from build123d import *

# Parameters (mm, degrees)
SKETCH1_W           = 10
SKETCH1_H           = 25
BOSS_EXTRUDE1_DEPTH = 8
SKETCH8_W           = 10
SKETCH8_H           = 2.3
BOSS_EXTRUDE4_DEPTH = 4
SKETCH9_W           = 10
SKETCH9_H           = 0.2
CUT_EXTRUDE3_DEPTH  = 4
SKETCH4_R           = 1.475
CUT_EXTRUDE2_DEPTH  = 8
LPATTERN1_COUNT     = 4
LPATTERN1_PITCH     = 5


with BuildPart() as part:
    # Sketch1 → Boss-Extrude1 (new body)
    with BuildSketch(Plane(origin=(0, 0, 0), x_dir=(1, 0, 0), z_dir=(0, 1, 0))):
        Rectangle(SKETCH1_W, SKETCH1_H)
    extrude(amount=BOSS_EXTRUDE1_DEPTH)

    # Sketch8 → Boss-Extrude4 (add)
    with BuildSketch(Plane(origin=(0, 8, 0), x_dir=(1, 0, 0), z_dir=(0, 1, 0))):
        with Locations((0, 11.35)):
            Rectangle(SKETCH8_W, SKETCH8_H)
        with Locations((0, -11.35)):
            Rectangle(SKETCH8_W, SKETCH8_H)
    extrude(amount=BOSS_EXTRUDE4_DEPTH)

    # Sketch9 → Cut-Extrude3 (cut)
    with BuildSketch(Plane(origin=(0, 8, 0), x_dir=(1, 0, 0), z_dir=(0, 1, 0))):
        with Locations((0, 10.1)):
            Rectangle(SKETCH9_W, SKETCH9_H)
        with Locations((0, -10.1)):
            Rectangle(SKETCH9_W, SKETCH9_H)
    extrude(amount=-CUT_EXTRUDE3_DEPTH, mode=Mode.SUBTRACT)

    # Sketch4 → Cut-Extrude2 (cut)
    with BuildSketch(Plane.XZ):
        with Locations(Location((0, 7.5, 0), (0, 0, 270))):
            Circle(SKETCH4_R)
    cut_extrude2 = extrude(amount=-CUT_EXTRUDE2_DEPTH, mode=Mode.SUBTRACT)

    # LPattern1: Cut-Extrude2 ×4
    with Locations(*[(0, 0, -i * LPATTERN1_PITCH) for i in range(1, LPATTERN1_COUNT)]):
        add(cut_extrude2, mode=Mode.SUBTRACT)


solid = part.part
CAD build for the part. Positions are in the model's coordinates, mm. A direction names the side the tool comes from. Round coordinates to 2 decimals unless told otherwise and drop trailing zeros. Loops run counter-clockwise (first coordinate to the right, second up) from the corner with the lowest first, then second, coordinate; pieces in that order, holes last.
(1) Cut at A-A (y = 7.5). Give the cut face in (x, z) (3 decimals).
(2) Cut at B-B (z = 2.5). Give the cut face in (x, y) (3 decimals).
(3) Drop a flat-ended pin along its axis: pin 1 (4.5 mm diameter, centred on x = 0, z = -2.5, fed in from +Y). Give the stop position or say it passes through.
(4) Two-plate mould, pull along X, no slides. Class faces 1 (the flat face through (-5, 5, 0)), 2 (the cylindrical face through (-0.565, 3.944, -3.863)), 3 (the flat face through (0, 6, -12.5)): +X half, -X half, draft (parallel to the pull), parting line (faces both ways), or undercut.
(5) Which spindle directions (+Z, -Z, +X, -X, +Y, -Y) get a long thin tool onto all of the face, cutting with end or side? Do faces 4 (the flat face through (0, 0, 0)), 5 (the flat face through (0, 6, -10)). Say none if no direction does.
(6) Cut at D-D (y = 1.5). Give the cut face in (x, z) (3 decimals), plus the area to 3 significant figures.
(7) Wall check: line 1 along Z through (x, y) = (-1.75, 4.75); line 2 along X through (y, z) = (2.5, 7.5) (3 decimals); line 3 along Z through (x, y) = (4.25, 8.25). Give the ranges that are in metal, low to high.
(8) Cut at C-C (x = 0). Give the cut face in (y, z) (3 decimals).
Findings below:
1. outline: (-5, -12.5) - (5, -12.5) - (5, -10.2) - (-5, -10.2) - close; (-5, -10) - (5, -10) - (5, 10) - (-5, 10) - close; (-5, 10.2) - (5, 10.2) - (5, 12.5) - (-5, 12.5) - close; hole circle Ø2.95 at (0, -7.5); hole circle Ø2.95 at (0, -2.5); hole circle Ø2.95 at (0, 2.5); hole circle Ø2.95 at (0, 7.5)
2. outline: (-5, 0) - (-1.475, 0) - (-1.475, 8) - (-5, 8) - close; (1.475, 0) - (5, 0) - (5, 8) - (1.475, 8) - close
3. pin 1: stops at y = 8
4. face 1: -X half
4. face 2: undercut
4. face 3: draft
5. face 4: +Z, -Z, +X, -X, -Y
5. face 5: +X, -X, +Y
6. outline: (-5, -12.5) - (5, -12.5) - (5, 12.5) - (-5, 12.5) - close; hole circle Ø2.95 at (0, -7.5); hole circle Ø2.95 at (0, -2.5); hole circle Ø2.95 at (0, 2.5); hole circle Ø2.95 at (0, 7.5)
6. area: 223 mm2
7. line 1: z = -12.5 to -10.2, -10 to 10, 10.2 to 12.5
7. line 2: x = -5 to -1.475, 1.475 to 5
7. line 3: z = -12.5 to -10.2, 10.2 to 12.5
8. outline: (0, -12.5) - (12, -12.5) - (12, -10.2) - (4, -10.2) - (4, -10) - (8, -10) - (8, -8.975) - (0, -8.975) - close; (0, -6.025) - (8, -6.025) - (8, -3.975) - (0, -3.975) - close; (0, -1.025) - (8, -1.025) - (8, 1.025) - (0, 1.025) - close; (0, 3.975) - (8, 3.975) - (8, 6.025) - (0, 6.025) - close; (0, 8.975) - (8, 8.975) - (8, 10) - (4, 10) - (4, 10.2) - (12, 10.2) - (12, 12.5) - (0, 12.5) - close
